Input: part model. Units: mm. Frame: model coordinates. Coordinates: 2 decimals unless noted, no trailing zeros. Order: outer loops, then holes, each group sorted by start corner. A loop starts at its lowest first (then second) coordinate and runs counter-clockwise, first axis right, second up. Notation, with made-up numbers: M -11.75,89.5 L 36.25,89.5 A12 ccw 36.25,96.5 Z; hole C 18,81.5 d4. An arc over 180 degrees is marked long. Answer in a Markdown table with one row per item.
from build123d import *

# Parameters (mm, degrees)
EXTRUDE_1_DEPTH          = 720
SKETCH_3_R               = 5
EXTRUDE_3_DEPTH          = 5
HOLE_WIZARD_1_AT_2_COUNT = 2
HOLE_WIZARD_1_AT_2_PITCH = 640
HOLE_WIZARD_1_AT_3_COUNT = 2
HOLE_WIZARD_1_AT_3_PITCH = 560
HOLE_WIZARD_1_AT_4_COUNT = 2
HOLE_WIZARD_1_AT_4_PITCH = 480
HOLE_WIZARD_1_AT_5_COUNT = 2
HOLE_WIZARD_1_AT_5_PITCH = 400
HOLE_WIZARD_1_AT_6_COUNT = 2
HOLE_WIZARD_1_AT_6_PITCH = 320
HOLE_WIZARD_1_AT_7_COUNT = 2
HOLE_WIZARD_1_AT_7_PITCH = 240
HOLE_WIZARD_1_AT_8_COUNT = 2
HOLE_WIZARD_1_AT_8_PITCH = 160
HOLE_WIZARD_1_AT_9_COUNT = 2
HOLE_WIZARD_1_AT_9_PITCH = 80
FILLET_1_R               = 0.5
FILLET_2_R               = 1
EXTRUDE_4_DEPTH          = 15
SKETCH_7_R               = 1.5
CUT_EXTRUDE_1_DEPTH      = 736.135021612


with BuildPart() as part:
    # ｽｹｯﾁ1 → ﾎﾞｽ - 押し出し1 (new body)
    with BuildSketch(Plane.XY.offset(720)):
        with BuildLine():
            Line((8.5, 3.408712153), (8.5, 2))
            Line((8.5, 2), (-8.5, 2))
            Line((-8.5, 2), (-8.5, 3.408712153))
            ThreePointArc((-8.5, 3.408712153), (-9.999347871, 5.642901666), (-8.603592403, 7.943230663))
            ThreePointArc((-8.603592403, 7.943230663), (-8.97237829, 8.349479447), (-9.5, 8.5))
            Line((-9.5, 8.5), (-12.5, 8.5))
            Line((-12.5, 8.5), (-12.5, 0))
            Line((-12.5, 0), (12.5, 0))
            Line((12.5, 0), (12.5, 8.5))
            Line((12.5, 8.5), (9.5, 8.5))
            ThreePointArc((9.5, 8.5), (8.97237829, 8.349479447), (8.603592403, 7.943230663))
            ThreePointArc((8.603592403, 7.943230663), (9.999347871, 5.642901666), (8.5, 3.408712153))
        make_face()
    extrude(amount=-EXTRUDE_1_DEPTH)

    # ｽｹｯﾁ3 → ﾎﾞｽ - 押し出し3 (add)
    with BuildSketch(Plane(origin=(0, 2, 0), x_dir=(-1, 0, 0), z_dir=(0, 1, 0))):
        with Locations(Location((0, 3, 0), (0, 0, 323.130102354))):
            Circle(SKETCH_3_R)
    extrude(amount=EXTRUDE_3_DEPTH)

    # ｽｹｯﾁ4 → 穴1 (revolve, cut)
    with BuildSketch(Plane(origin=(0, 2, 40), x_dir=(0, 0, 1), z_dir=(1, 0, 0))):
        Polygon((0, 0), (0, 2), (2.25, 2), (4.25, 0), align=None)
    hole_wizard_1 = revolve(axis=Axis((0, -108, 40), (0, 1, 0)), mode=Mode.SUBTRACT)

    # 穴1 at 2: 穴1 ×2
    with Locations(*[(0, 0, i * HOLE_WIZARD_1_AT_2_PITCH) for i in range(1, HOLE_WIZARD_1_AT_2_COUNT)]):
        add(hole_wizard_1, mode=Mode.SUBTRACT)

    # 穴1 at 3: 穴1 ×2
    with Locations(*[(0, 0, i * HOLE_WIZARD_1_AT_3_PITCH) for i in range(1, HOLE_WIZARD_1_AT_3_COUNT)]):
        add(hole_wizard_1, mode=Mode.SUBTRACT)

    # 穴1 at 4: 穴1 ×2
    with Locations(*[(0, 0, i * HOLE_WIZARD_1_AT_4_PITCH) for i in range(1, HOLE_WIZARD_1_AT_4_COUNT)]):
        add(hole_wizard_1, mode=Mode.SUBTRACT)

    # 穴1 at 5: 穴1 ×2
    with Locations(*[(0, 0, i * HOLE_WIZARD_1_AT_5_PITCH) for i in range(1, HOLE_WIZARD_1_AT_5_COUNT)]):
        add(hole_wizard_1, mode=Mode.SUBTRACT)

    # 穴1 at 6: 穴1 ×2
    with Locations(*[(0, 0, i * HOLE_WIZARD_1_AT_6_PITCH) for i in range(1, HOLE_WIZARD_1_AT_6_COUNT)]):
        add(hole_wizard_1, mode=Mode.SUBTRACT)

    # 穴1 at 7: 穴1 ×2
    with Locations(*[(0, 0, i * HOLE_WIZARD_1_AT_7_PITCH) for i in range(1, HOLE_WIZARD_1_AT_7_COUNT)]):
        add(hole_wizard_1, mode=Mode.SUBTRACT)

    # 穴1 at 8: 穴1 ×2
    with Locations(*[(0, 0, i * HOLE_WIZARD_1_AT_8_PITCH) for i in range(1, HOLE_WIZARD_1_AT_8_COUNT)]):
        add(hole_wizard_1, mode=Mode.SUBTRACT)

    # 穴1 at 9: 穴1 ×2
    with Locations(*[(0, 0, i * HOLE_WIZARD_1_AT_9_PITCH) for i in range(1, HOLE_WIZARD_1_AT_9_COUNT)]):
        add(hole_wizard_1, mode=Mode.SUBTRACT)

    # ﾌｨﾚｯﾄ1
    fillet_1_edges = [part.edges().sort_by_distance(p)[0] for p in [
        (-8.5, 2, 360),
        (8.5, 2, 360),
    ]]
    fillet(fillet_1_edges, radius=FILLET_1_R)

    # ﾌｨﾚｯﾄ2
    fillet_2_edges = [part.edges().sort_by_distance(p)[0] for p in [
        (12.5, 8.5, 360),
        (12.5, 0, 360),
        (-12.5, 0, 360),
        (-12.5, 8.5, 360),
    ]]
    fillet(fillet_2_edges, radius=FILLET_2_R)

    # ｽｹｯﾁ6 → ﾎﾞｽ - 押し出し4 (add)
    with BuildSketch(Plane.XY.offset(720)):
        with BuildLine():
            ThreePointArc((-12.5, 1), (-12.207106781, 0.292893219), (-11.5, 0))
            Line((-11.5, 0), (11.5, 0))
            ThreePointArc((11.5, 0), (12.207106781, 0.292893219), (12.5, 1))
            Line((12.5, 1), (12.5, 7.5))
            ThreePointArc((12.5, 7.5), (12.207106781, 8.207106781), (11.5, 8.5))
            Line((11.5, 8.5), (9.5, 8.5))
            ThreePointArc((9.5, 8.5), (8.97237829, 8.349479447), (8.603592403, 7.943230663))
            ThreePointArc((8.603592403, 7.943230663), (9.999347871, 5.642901666), (8.5, 3.408712153))
            Line((8.5, 3.408712153), (8.5, 2.5))
            ThreePointArc((8.5, 2.5), (8.353553391, 2.146446609), (8, 2))
            Line((8, 2), (-8, 2))
            ThreePointArc((-8, 2), (-8.353553391, 2.146446609), (-8.5, 2.5))
            Line((-8.5, 2.5), (-8.5, 3.408712153))
            ThreePointArc((-8.5, 3.408712153), (-9.999347871, 5.642901666), (-8.603592403, 7.943230663))
            ThreePointArc((-8.603592403, 7.943230663), (-8.97237829, 8.349479447), (-9.5, 8.5))
            Line((-9.5, 8.5), (-11.5, 8.5))
            ThreePointArc((-11.5, 8.5), (-12.207106781, 8.207106781), (-12.5, 7.5))
            Line((-12.5, 7.5), (-12.5, 1))
        make_face()
    extrude(amount=EXTRUDE_4_DEPTH)

    # ｽｹｯﾁ7 → ｶｯﾄ - 押し出し1 (cut, through all)
    with BuildSketch(Plane(origin=(0, 2, 0), x_dir=(1, 0, 0), z_dir=(0, 1, 0))):
        with Locations(Location((0, -732, 0), (0, 0, 270))):
            Circle(SKETCH_7_R)
    extrude(amount=-CUT_EXTRUDE_1_DEPTH, mode=Mode.SUBTRACT)


solid = part.part
1) Contact query for flat-ended pins moving along their axis: pin 1 (1.5 mm diameter, centred on x = 1, y = 5.5, fed in from +Z); pin 2 (13 mm diameter, centred on x = -0.5, z = 342.5, fed in from +Y); pin 3 (3 mm diameter, centred on x = -0.5, z = 3.5, fed in from +Y). Output: stop coordinate, or through.
Resolved:
| item | result |
|---|---|
| pin 1 | stops at z = 7.99 |
| pin 2 | stops at y = 2 |
| pin 3 | stops at y = 7 |
2) Mould query, pull axis X, two halves, no side actions, for faces 1 (the face through (-3, 0, 362)), 2 (the face through (4, 2, 362)). Classes: +X half, -X half, draft (parallel to the pull), parting line (faces both ways), or undercut.
Resolved:
| item | result |
|---|---|
| face 1 | draft |
| face 2 | undercut |
3) Cut plane A-A, the plane y = 5. Output: boundary loops of the cut face in (x, z).
Resolved:
| item | result |
|---|---|
| outline | M -12.5,0 L -9.9,0 L -9.9,735 L -12.5,735 Z; C 0,3 d10; M 9.9,0 L 12.5,0 L 12.5,735 L 9.9,735 Z |
4) Cut plane B-B, the plane z = 632. Output: boundary loops of the cut face in (x, y), and give its area (3 significant figures).
Resolved:
| item | result |
|---|---|
| outline | M -12.5,1 A1 ccw -11.5,0 L 11.5,0 A1 ccw 12.5,1 L 12.5,7.5 A1 ccw 11.5,8.5 L 9.5,8.5 A1 ccw 8.6,7.94 A2.5 cw 8.5,3.41 L 8.5,2.5 A0.5 cw 8,2 L -8,2 A0.5 cw -8.5,2.5 L -8.5,3.41 A2.5 cw -8.6,7.94 A1 ccw -9.5,8.5 L -11.5,8.5 A1 ccw -12.5,7.5 Z |
| area | 90.9 mm2 |
5) Material intervals for probe 1 along X at (y, z) = (0.8, 732); probe 2 along X at (y, z) = (7.25, 99.5); probe 3 along Z at (x, y) = (-10.5, 7), sorted ascending.
Resolved:
| item | result |
|---|---|
| probe 1 | x = -12.48 to -1.5, 1.5 to 12.48 |
| probe 2 | x = -12.5 to -9.46, 9.46 to 12.5 |
| probe 3 | z = 0 to 735 |
